Geometry: final body of the model. Coordinates: model frame, mm. A direction names the side the tool comes from. Round coordinates to 2 decimals unless told otherwise and drop trailing zeros. Loops run counter-clockwise (first coordinate to the right, second up) from the corner with the lowest first, then second, coordinate; pieces in that order, holes last. Notation, with made-up numbers: (56.25, -33.5) -> (65.25, -33.5) arc R19 ccw to (65.25, -8.5) -> close; hole circle Ø10 at (67, -10.75). An arc over 180 degrees is marked (long way). Answer in a Markdown table with one row per item.
```python
from build123d import *

# Parameters (mm, degrees)
F0_W     = 150
F0_H     = 100
F1_DEPTH = 101.6
F2_R     = 20
F3_T     = -2.54


with BuildPart() as f1:
    # F0 (on Front) → F1 (new body)
    with BuildSketch(Plane.XZ):
        with Locations((-35.558602, -17.734206)):
            Rectangle(F0_W, F0_H)
    extrude(amount=F1_DEPTH)

    # F2
    f2_edges = [f1.edges().sort_by_distance(p)[0] for p in [
        (-35.558602, -101.6, -67.734206),
    ]]
    fillet(f2_edges, radius=F2_R)

    # F3
    f3_openings = [f1.faces().sort_by_distance(p)[0] for p in [
        (-35.558602, 0, -17.734206),
        (-35.558602, -50.8, 32.265794),
    ]]
    offset(amount=F3_T, openings=f3_openings)


solid = f1.part
```
Item 1: Cut plane A-A (x = -51.5). Output: boundary loops of the cut face in (y, z), then the cut area to 3 significant figures.
Answer:
| item | result |
|---|---|
| outline | (-101.6, -47.73) arc R20 ccw to (-81.6, -67.73) -> (0, -67.73) -> (0, -65.19) -> (-81.6, -65.19) arc R17.46 cw to (-99.06, -47.73) -> (-99.06, 32.27) -> (-101.6, 32.27) -> close |
| area | 485 mm² |
Item 2: Pin query (flat end, axial travel): pin 1 Ø2 at (x, y) = (-57.5, -87) entering from -Z; pin 2 Ø12 at (x, z) = (-43, -30) entering from +Y; pin 3 Ø6 at (x, y) = (-19, -59) entering from +Z. Return the tip coordinate at first contact, or that it passes through.
Answer:
| item | result |
|---|---|
| pin 1 | stops at z = -67.24 |
| pin 2 | stops at y = -99.06 |
| pin 3 | stops at z = -65.19 |
Item 3: Cut plane B-B (y = -19). Output: boundary loops of the cut face in (x, z), then the cut area to 3 significant figures.
Answer:
| item | result |
|---|---|
| outline | (-110.56, -67.73) -> (39.44, -67.73) -> (39.44, 32.27) -> (36.9, 32.27) -> (36.9, -65.19) -> (-108.02, -65.19) -> (-108.02, 32.27) -> (-110.56, 32.27) -> close |
| area | 876 mm² |
Item 4: Line query: probe 1 along X at (y, z) = (-73, 19.5); probe 2 along Z at (x, y) = (-62.5, -12.5); probe 3 along Y at (x, z) = (-1.5, 1). Output: solid intervals per line, ascending. Write a range as [from, to].
Answer:
| item | result |
|---|---|
| probe 1 | x = [-110.56, -108.02], [36.9, 39.44] |
| probe 2 | z = [-67.73, -65.19] |
| probe 3 | y = [-101.6, -99.06] |
Item 5: Draft query along X for faces 3 (the face through (-110.559, -50, -18)), 4 (the face through (-37, -101.6, -7)), 5 (the face through (-34.544, -93.81, -60.215)). Return one class per face: pulls with the +X half, pulls with the -X half, needs draft (parallel to the pull), parting line crosses it, or undercut.
Answer:
| item | result |
|---|---|
| face 3 | pulls with the -X half |
| face 4 | needs draft |
| face 5 | undercut |
Item 6: Reachability of faces 1 (the face through (39.441, -50, -18)), 2 (the face through (36.901, -49, -17)) from +Z, -Z, +X, -X, +Y, -Y: full face, straight path, thin tool, end or side. Return the list, or none.
Answer:
| item | result |
|---|---|
| face 1 | +Z, -Z, +X, +Y, -Y |
| face 2 | +Z, +Y |
